Here's how the part is built. I have some questions about the finished solid (model axes, mm). A direction names the side the tool comes from. Round coordinates to 2 decimals unless told otherwise and drop trailing zeros. Loops run counter-clockwise (first coordinate to the right, second up) from the corner with the lowest first, then second, coordinate; pieces in that order, holes last. Notation, with made-up numbers: (-18, 30) - (-9, 30) arc R8 ccw to (-9, 35) - close; hole circle Ø2 at (-26.75, 89.5). An arc over 180 degrees is marked (long way). Answer as a JSON object with one key per item and string values. Group by question number.
1) I want a section at B-B, the plane z = -22.5. Please give me the cut outline in (x, y), then the cut area to 3 significant figures.
2) Which directions (+Z, -Z, +X, -X, +Y, -Y) give clear straight access to the entire face, cutting with the end or side of a thin tool? Please do faces 1 (the face through (-95, 35, -18)), 2 (the face through (-135, 33, -8)).
3) If I drill on line 1 along X through (y, z) = (55, 16); line 2 along Z through (x, y) = (6, 14.5); line 3 along Z through (x, y) = (92, 39), over which ranges is the centre line in solid material (lowest first)? Write a range as [from, to].
4) I want a section at C-C, the plane y = 60. Please give me the cut outline in (x, z), then the cut area to 3 significant figures.
5) I want a section at A-A, the plane y = 34. Please give me the cut outline in (x, z), then the cut area to 3 significant figures.
6) Will these pins go through, and if not, where does the flat tip stop? P1, Ø10, axis at x = -16, y = 17.5, coming from the +Z side; P2, Ø4, axis at x = -63.5, y = 5.5, coming from the +Z side; P3, Ø8, axis at x = 36, y = 46.5, coming from the -Z side.
7) I want a section at D-D, the plane x = -69. Please give me the cut outline in (y, z).
from build123d import *

# Parameters (mm, degrees)
BOSS_EXTRUDE1_DEPTH      = 70
BOSS_EXTRUDE1_DEPTH_BACK = 2
SKETCH1_W                = 270
SKETCH1_H                = 110
CUT_EXTRUDE3_DEPTH       = 331
SKETCH18_W               = 270
SKETCH18_H               = 72
BOSS_EXTRUDE3_DEPTH      = 30
CUT_EXTRUDE16_DEPTH      = 292.590466236
CUT_EXTRUDE16_DEPTH_BACK = 292.590466236
CUT_EXTRUDE17_DEPTH      = 176.025712397
CUT_EXTRUDE17_DEPTH_BACK = 176.025712397


with BuildPart() as part:
    # Sketch1 → Boss-Extrude1 (new, two sides: drawn at the far end of the back side and taken through both)
    with BuildSketch(Plane(origin=(0, 0, 0), x_dir=(1, 0, 0), z_dir=(0, 1, 0)).offset(-BOSS_EXTRUDE1_DEPTH_BACK)):
        Rectangle(SKETCH1_W, SKETCH1_H)
    extrude(amount=BOSS_EXTRUDE1_DEPTH + BOSS_EXTRUDE1_DEPTH_BACK)

    # Sketch2 → Cut-Extrude3 (cut)
    with BuildSketch(Plane(origin=(0, 70, 0), x_dir=(1, 0, 0), z_dir=(0, 1, 0))):
        Polygon((-95, 55), (-95, -20), (0, -20), (95, -20), (95, 55), align=None)
    extrude(amount=-CUT_EXTRUDE3_DEPTH, mode=Mode.SUBTRACT)

    # Sketch18 → Boss-Extrude3 (add)
    with BuildSketch(Plane.XY.offset(55)):
        with Locations((0, 34)):
            Rectangle(SKETCH18_W, SKETCH18_H)
    extrude(amount=BOSS_EXTRUDE3_DEPTH)

    # Sketch19 → Cut-Extrude16 (cut, two sides: drawn at the far end of the back side and taken through both)
    with BuildSketch(Plane(origin=(135, 0, 0), x_dir=(0, 0, -1), z_dir=(1, 0, 0)).offset(-CUT_EXTRUDE16_DEPTH_BACK)):
        with BuildLine():
            Line((-379.944046873, -39.064261373), (-85, 40))
            Line((-85, 40), (25.116182189, 69.51832628))
            ThreePointArc((25.116182189, 69.51832628), (45.85724684, 64.327382716), (55, 45))
            Line((55, 45), (55, -260.357410606))
            Line((55, -260.357410606), (331.938852434, 283.956345293))
            Line((331.938852434, 283.956345293), (-103.005194439, 505.249494526))
            Line((-103.005194439, 505.249494526), (-379.944046873, -39.064261373))
        make_face()
    extrude(amount=CUT_EXTRUDE16_DEPTH + CUT_EXTRUDE16_DEPTH_BACK, mode=Mode.SUBTRACT)

    # Sketch21 → Cut-Extrude17 (cut, two sides: drawn at the far end of the back side and taken through both)
    with BuildSketch(Plane.XZ.offset(2).offset(-CUT_EXTRUDE17_DEPTH_BACK)):
        with BuildLine():
            ThreePointArc((3.953760881, 85), (69.754776005, 75.238802072), (130.348831285, 47.79039518))
            ThreePointArc((130.348831285, 47.79039518), (133.760374217, 44.16356592), (135, 39.341134628))
            Line((135, 39.341134628), (135, 85))
            Line((135, 85), (3.953760881, 85))
        make_face()
        with BuildLine():
            ThreePointArc((-130.348831285, 47.79039518), (-69.754776005, 75.238802072), (-3.953760881, 85))
            Line((-3.953760881, 85), (-135, 85))
            Line((-135, 85), (-135, 39.341134628))
            ThreePointArc((-135, 39.341134628), (-133.760374217, 44.16356592), (-130.348831285, 47.79039518))
        make_face()
    extrude(amount=CUT_EXTRUDE17_DEPTH + CUT_EXTRUDE17_DEPTH_BACK, mode=Mode.SUBTRACT)


solid = part.part
Outcome:
{
 "1": {"outline": "(-135, -2) - (-95, -2) - (-95, 68.82) - (-135, 68.82) - close; (95, -2) - (135, -2) - (135, 68.82) - (95, 68.82) - close", "area": "5,670 mm^2"},
 "2": {"face 1": "-Z, +Y, -Y", "face 2": "+Z, -Z, -X, +Y, -Y"},
 "3": {"line 1": "[-135, -95], [95, 135]", "line 2": "[20, 84.97]", "line 3": "[20, 67.48]"},
 "4": {"outline": "(-135, -50) - (-95, -50) - (-95, 10.39) - (-135, 10.39) - close; (95, -50) - (135, -50) - (135, 10.39) - (95, 10.39) - close", "area": "4,830 mm^2"},
 "5": {"outline": "(-135, -55) - (-95, -55) - (-95, 20) - (95, 20) - (95, -55) - (135, -55) - (135, 39.34) arc R10 ccw to (130.35, 47.79) arc R240 ccw to (3.95, 85) - (-3.95, 85) arc R240 ccw to (-130.35, 47.79) arc R10 ccw to (-135, 39.34) - close", "area": "20,100 mm^2"},
 "6": {"P1": "z = 84.84", "P2": "z = 77.51", "P3": "z = 20"},
 "7": {"outline": "(-2, 20) - (57.42, 20) - (42.56, 75.46) - (-2, 75.46) - close"}
}
